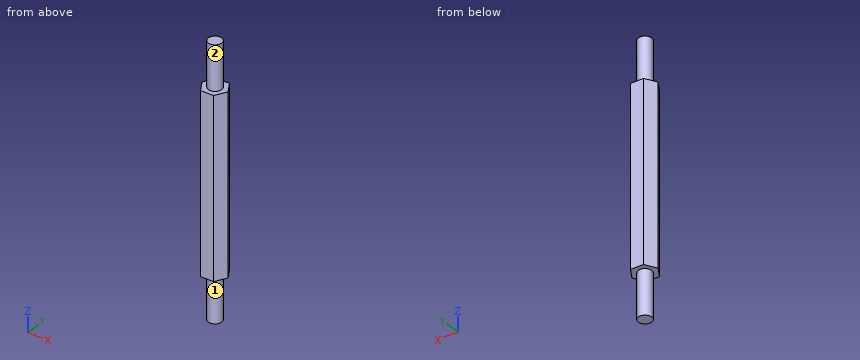
```python
from build123d import *

# Parameters (mm, degrees)
BOSS_EXTRU_1_DEPTH = 40
ESQUISSE2_R        = 1.5
BOSS_EXTRU_2_DEPTH = 10
ESQUISSE3_R        = 1.5
BOSS_EXTRU_3_DEPTH = 10


with BuildPart() as part:
    # Esquisse1 → Boss.-Extru.1 (new body)
    with BuildSketch(Plane.XY):
        Polygon((1.470451141, -2.484171245), (2.886580976, 0.03136242), (1.416129835, 2.515533666), (-1.470451141, 2.484171245), (-2.886580976, -0.03136242), (-1.416129835, -2.515533666), align=None)
    extrude(amount=BOSS_EXTRU_1_DEPTH)

    # Esquisse2 → Boss.-Extru.2 (add)
    with BuildSketch(Plane.XY.offset(40)):
        Circle(ESQUISSE2_R)
    extrude(amount=BOSS_EXTRU_2_DEPTH)

    # Esquisse3 → Boss.-Extru.3 (add)
    with BuildSketch(Plane(origin=(0, 0, 0), x_dir=(-1, 0, 0), z_dir=(0, 0, -1))):
        Circle(ESQUISSE3_R)
    extrude(amount=BOSS_EXTRU_3_DEPTH)


solid = part.part
```
Model file for the job. Use its own axes, mm. Face numbers are marked on the shaded views. A direction names the side the tool comes from. Give positions to 0.01 mm unless a question says otherwise; leave off trailing zeros. Order: outer loops, then holes, each group sorted by start corner. A loop starts at its lowest first (then second) coordinate and runs counter-clockwise, first axis right, second up.
1) Saw through at A-A, the plane z = 21. Write the cut outline in (x, y), then the cut area to 3 significant figures.
2) 3-axis set-ups, long thin cutter, end or side, ignore diameter. For the marked faces 1 and 2: which of +Z, -Z, +X, -X, +Y, -Y reach the whole face in a straight line?
3) Saw through at D-D, the plane z = -4.5. Write the cut outline in (x, y).
4) Saw through at B-B, the plane y = 0.65. Write the cut outline in (x, z).
5) Pin check, flat tip, straight feed: pin 1 (1.5 mm diameter, centred on y = -1.5, z = 25.5, fed in from -X). Stop position of the tip, or through.
6) Wall check: probe 1 along Y at (x, z) = (0.6, 18.5); probe 2 along Z at (x, y) = (-1, 1.3); probe 3 along Y at (x, z) = (-0.25, 41). Give the ranges that are in metal, low to high.
7) Saw through at C-C, the plane x = 0.2. Write the cut outline in (y, z), then the cut area to 3 significant figures.
Computed:
1. outline: (-2.89, -0.03) - (-1.42, -2.52) - (1.47, -2.48) - (2.89, 0.03) - (1.42, 2.52) - (-1.47, 2.48) - close
1. area: 21.7 mm2
2. face 1: -Z
2. face 2: +Z
3. outline: circle Ø3 at (0, 0)
4. outline: (-2.5, 0) - (-1.35, 0) - (-1.35, -10) - (1.35, -10) - (1.35, 0) - (2.52, 0) - (2.52, 40) - (1.35, 40) - (1.35, 50) - (-1.35, 50) - (-1.35, 40) - (-2.5, 40) - close
5. pin 1: stops at x = -2.46
6. probe 1: y = -2.49 to 2.51
6. probe 2: z = 0 to 40
6. probe 3: y = -1.48 to 1.48
7. outline: (-2.5, 0) - (-1.49, 0) - (-1.49, -10) - (1.49, -10) - (1.49, 0) - (2.5, 0) - (2.5, 40) - (1.49, 40) - (1.49, 50) - (-1.49, 50) - (-1.49, 40) - (-2.5, 40) - close
7. area: 259 mm2
